```python
from build123d import *

# Parameters (mm, degrees)
BOSS_EXTRUDE1_DEPTH = 3
FILLET1_R           = 4
FILLET2_R           = 1
FILLET3_R           = 1
SKETCH2_W           = 68.766076313
SKETCH2_H           = 3.02
CUT_EXTRUDE3_DEPTH  = 10
SKETCH3_W           = 3.5
SKETCH3_H           = 3.02
BOSS_EXTRUDE2_DEPTH = 3


with BuildPart() as part:
    # Sketch1 → Boss-Extrude1 (new body)
    with BuildSketch(Plane.XY):
        with BuildLine():
            Line((0, 35), (0, 40.154947939))
            Line((0, 40.154947939), (1.79, 40.154947939))
            Line((1.79, 40.154947939), (1.79, 35))
            Line((1.79, 35), (6.75, 35))
            Line((6.75, 35), (6.75, 50))
            Line((6.75, 50), (0, 50))
            Line((0, 50), (0, 45))
            ThreePointArc((0, 45), (-44.925333381, 2.591219899), (-5.173840791, -44.701581308))
            Line((-5.173840791, -44.701581308), (-11.99982612, -32.878627908))
            ThreePointArc((-11.99982612, -32.878627908), (-34.465576861, 6.092947695), (0, 35))
        make_face()
    extrude(amount=BOSS_EXTRUDE1_DEPTH)

    # Fillet1
    fillet1_edges = [part.edges().sort_by_distance(p)[0] for p in [
        (0, 45, 1.5),
    ]]
    fillet(fillet1_edges, radius=FILLET1_R)

    # Fillet2
    fillet2_edges = [part.edges().sort_by_distance(p)[0] for p in [
        (-5.173840791, -44.701581308, 1.5),
    ]]
    fillet(fillet2_edges, radius=FILLET2_R)

    # Fillet3
    fillet3_edges = [part.edges().sort_by_distance(p)[0] for p in [
        (-11.99982612, -32.878627908, 1.5),
    ]]
    fillet(fillet3_edges, radius=FILLET3_R)

    # Sketch2 → Cut-Extrude3 (cut)
    with BuildSketch(Plane.XY.offset(3)):
        with Locations((0.383038156, -22.906441492)):
            Rectangle(SKETCH2_W, SKETCH2_H)
    extrude(amount=-CUT_EXTRUDE3_DEPTH, mode=Mode.SUBTRACT)

    # Sketch3 → Boss-Extrude2 (add)
    with BuildSketch(Plane.XY.offset(3)):
        with Locations((-32.25, -22.906441492)):
            Rectangle(SKETCH3_W, SKETCH3_H)
    extrude(amount=-BOSS_EXTRUDE2_DEPTH)


solid = part.part
```
Model file for the job. Use its own axes, mm. A direction names the side the tool comes from. Give positions to 0.01 mm unless a question says otherwise; leave off trailing zeros. Write each loop counter-clockwise with the first axis right and the second up, starting at its lowest first coordinate (ties: lowest second). Pieces come first, ordered by that corner, then holes. Notation, with made-up numbers: (62.5, 47.5) -> (95.5, 47.5) arc R24 ccw to (95.5, 68.5) -> close; hole circle Ø10 at (74.5, 4). An arc over 180 degrees is marked (long way). Use CSV: the item, a comma, the result in double quotes. Start each with the question number.
1) Drill centre lines: L1, parallel to X at y = -1, z = 1.3; L2, parallel to Y at x = -9, z = 1.2; L3, parallel to Y at x = -11, z = 1.2. Where is each one in solid material? Low to high.
2) Two-plate mould, pull along Y, no slides. Class faces 1 (the cylindrical face through (-1.03, 46.16, 1.52)), 2 (the flat face through (-28, -24.416, 2)), 3 (the flat face through (6.75, 42, 1)): released by +Y, released by -Y, zero draft, split by the parting line, or undercut.
3) Tool access for faces 4 (the flat face through (-35, 7, 0)), 5 (the flat face through (-30.5, -23, 2)), 6 (the flat face through (-35, 7, 3)), 7 (the flat face through (4, 35, 1)), 8 (the flat face through (1, 40.155, 1)): list every direction of +Z, -Z, +X, -X, +Y, -Y with a clear straight run to the whole face (end or side of a thin tool).
4) Cut at A-A on z = 0.8. List the corners of the cut face in (x, y).
5) Cut at C-C on x = -37.5. List the corners of the cut face in (y, z).
6) Cut at B-B on y = 32. List the corners of the cut face in (x, z).
7) Pin check, flat tips, straight feed: P1, Ø0.9, axis at y = -22.5, z = 1.5, coming from the +X side; P2, Ø1.5, axis at y = -29.5, z = 2.5, coming from the +X side; P3, Ø0.9, axis at y = 37, z = 1.5, coming from the -X side. Stop position of each tip, or through.
Final values:
1,L1,"x = -44.99 to -34.99"
1,L2,"y = -44.09 to -38.07, 33.82 to 44.09"
1,L3,"y = -43.63 to -34.61, 33.23 to 43.63"
2,face 1,"released by +Y"
2,face 2,"undercut"
2,face 3,"zero draft"
3,face 4,"-Z, +X, -X, +Y, -Y"
3,face 5,"+Z, -Z, +X"
3,face 6,"+Z, +X, -X, +Y, -Y"
3,face 7,"+Z, -Z, +X, -Y"
3,face 8,"+Z, -Z, -Y"
4,outline,"(-30.5, -24.42) -> (-30.5, -21.4) -> (-27.7, -21.4) arc R35 cw to (0, 35) -> (0, 40.15) -> (1.79, 40.15) -> (1.79, 35) -> (6.75, 35) -> (6.75, 50) -> (0, 50) -> (0, 48.84) arc R4 cw to (-3.67, 44.85) arc R45 ccw to (-7.22, -44.42) arc R1 ccw to (-6.2, -42.93) -> (-11.82, -33.19) arc R1 ccw to (-12.33, -32.76) arc R35 cw to (-25.08, -24.42) -> close"
5,outline,"(-24.87, 0) -> (24.87, 0) -> (24.87, 3) -> (-24.87, 3) -> close"
6,outline,"(-31.64, 0) -> (-14.18, 0) -> (-14.18, 3) -> (-31.64, 3) -> close"
7,P1,"stops at x = -30.5"
7,P2,"stops at x = -17.61"
7,P3,"stops at x = -26.25"
